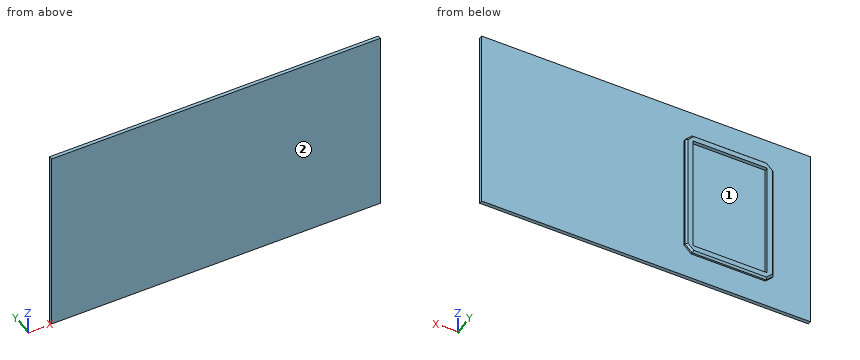
Autodesk Inventor part; units mm, degrees
ref_plane "YZ Plane" through (0, 0, 0) normal (1, 0, 0) x (0, 1, 0)
ref_plane "XZ Plane" through (0, 0, 0) normal (0, 1, 0) x (-1, 0, 0)
ref_plane "XY Plane" through (0, 0, 0) normal (0, 0, 1) x (1, 0, 0)
sketch "Sketch1" plane through (0, 0, 0) normal (0, 1, 0) x (-1, 0, 0)
  line L0 (0, 0) -> (-609.6, 0)
  line L1 (-609.6, 0) -> (-609.6, -342.9)
  line L2 (-609.6, -342.9) -> (0, -342.9)
  line L3 (0, -342.9) -> (0, 0)
  dimension "d0" = 609.6
  dimension "d1" = 342.9
  dimension "d2" = 609.6
extrude "Extrusion1" add sketch "Sketch1" along normal blind 6.35
sketch "Sketch2" plane through (0, 0, 0) normal (0, 1, 0) x (-1, 0, 0)
  line L0 (-609.6, -342.9) -> (0, -342.9)
  line L1 (0, 0) -> (-609.6, 0)
  line L2 (-609.6, -342.9) -> (-603.25, -342.9)
  line L3 (-603.25, -342.9) -> (-603.25, 0)
  line L4 (-603.25, 0) -> (-609.6, 0)
  line L5 (-609.6, 0) -> (-609.6, -342.9)
  dimension "d5" = 6.35
extrude "Extrusion2" cut sketch "Sketch2" along normal blind 231.775
sketch "Sketch3" plane through (0, 6.35, 0) normal (0, 1, 0) x (1, 0, 0)
  line L0 (603.25, 0) -> (603.25, 342.9)
  line L1 (0, 342.9) -> (0, 0)
  dimension "d8" = 603.25
sketch "Sketch4" plane through (0, 6.35, 0) normal (0, 1, 0) x (1, 0, 0)
  line L0 (603.25, 342.9) -> (0, 342.9)
  line L1 (0, 0) -> (603.25, 0)
  line L2 (0, 342.9) -> (0, 0)
  line L3 (0, 0) -> (301.625, 0)
  line L4 (301.625, 0) -> (301.625, 342.9)
  line L5 (301.625, 0) -> (452.4375, 0)
  line L6 (82.8675, 171.45) -> (82.8675, 280.162)
  line L7 (82.8675, 280.162) -> (150.8125, 280.162)
  line L8 (82.8675, 171.45) -> (82.8675, 62.738)
  line L9 (82.8675, 62.738) -> (150.8125, 62.738)
  line L10 (218.7575, 280.162) -> (150.8125, 280.162)
  line L11 (218.7575, 171.45) -> (218.7575, 280.162)
  line L12 (218.7575, 171.45) -> (218.7575, 62.738)
  line L13 (218.7575, 62.738) -> (150.8125, 62.738)
  line L14 (218.7575, 280.162) -> (218.7575, 292.862)
  line L15 (218.7575, 292.862) -> (82.8675, 292.862)
  line L16 (82.8675, 292.862) -> (82.8675, 280.162)
  line L17 (87.7385, 280.162) -> (75.0385, 280.162)
  line L18 (77.9965, 62.738) -> (87.7385, 62.738)
  line L19 (82.8675, 280.162) -> (70.1675, 280.162)
  line L20 (70.1675, 280.162) -> (70.1675, 62.738)
  line L21 (70.1675, 62.738) -> (82.8675, 62.738)
  line L22 (82.8675, 62.738) -> (82.8675, 50.038)
  line L23 (82.8675, 50.038) -> (218.7575, 50.038)
  line L24 (218.7575, 50.038) -> (218.7575, 62.738)
  line L25 (218.7575, 62.738) -> (231.4575, 62.738)
  line L26 (231.4575, 62.738) -> (231.4575, 280.162)
  line L27 (231.4575, 280.162) -> (218.7575, 280.162)
  line L28 (231.4575, 62.738) -> (218.7575, 50.038)
  line L29 (82.8675, 50.038) -> (70.1675, 62.738)
  line L30 (70.1675, 62.738) -> (70.1675, 280.162)
  line L31 (82.8675, 292.862) -> (70.1675, 280.162)
  line L32 (218.7575, 292.862) -> (231.4575, 280.162)
  dimension "d9" = 342.9
  dimension "d10" = 301.625
  dimension "d11" = 150.8125
extrude "Extrusion3" add sketch "Sketch4" along normal blind 6.35 contours L8 L18 L21 L20 L19 L17 L6 | L16 L15 L14 L10 L7 | L17 L19 L31 L16 | L22 L29 L21 L18 | L9 L13 L24 L23 L22 | L32 L27 L14 | L24 L25 L28 | L27 L26 L25 L12 L11
chamfer "Chamfer1" distance 3.175 angle 45 8 edges at (70.1675, 12.7, -171.45) (76.5175, 12.7, -286.512) (150.8125, 12.7, -292.862) (225.1075, 12.7, -286.512) (231.4575, 12.7, -171.45) (225.1075, 12.7, -56.388) (150.8125, 12.7, -50.038) (76.5175, 12.7, -56.388)
properties part number "UpperHalfofFrontBack_Ocampo"
Check sheet for the modelled part. Datum: model origin and axes. Units: mm. Face numbers are marked on the shaded views. A direction names the side the tool comes from. Coordinates: 2 decimals unless noted, no trailing zeros. Order: outer loops, then holes, each group sorted by start corner. A loop starts at its lowest first (then second) coordinate and runs counter-clockwise, first axis right, second up. Notation, with made-up numbers: (84, -8) -> (140, -8) arc R20 ccw to (140, -3) -> close; hole circle Ø8 at (-22.75, 75). An arc over 180 degrees is marked (long way). Write item = value, one per line. Start each with the question number.
1) Go/stop test with flat-tipped pins: P1, Ø2.5, axis at x = 175.5, y = 8, coming from the +Z side; P2, Ø3, axis at y = 9.5, z = -143.5, coming from the +X side; P3, Ø2.5, axis at y = 8, z = -119, coming from the -X side. Record where each tip stops, or that it passes through.
2) Cross-section at C-C (z = -314). Enter the section's corners in (x, y), then the cut area to 3 significant figures.
3) Cross-section at A-A (x = 110). Enter the section's corners in (y, z) (3 decimals).
4) Access from +Z, -Z, +X, -X, +Y, -Y to the whole of each face (thin tool, end or side, straight path). Record for the marked faces 1 and 2.
5) Material ranges on L1, parallel to X at y = 6.75, z = -164.5; L2, parallel to Y at x = 59.5, z = -94; L3, parallel to X at y = 11, z = -218.5, recorded low to high.
6) Cross-section at D-D (x = 342.5). Enter the section's corners in (y, z), then the cut area to 3 significant figures.
Ans:
q1.P1 = -50.04
q1.P2 = 231.46
q1.P3 = 70.17
q2.outline = (0, 0) -> (603.25, 0) -> (603.25, 6.35) -> (0, 6.35) -> close
q2.area = 3,830 mm²
q3.outline = (0, -342.9) -> (6.35, -342.9) -> (6.35, -292.862) -> (9.525, -292.862) -> (12.7, -289.687) -> (12.7, -280.162) -> (6.35, -280.162) -> (6.35, -62.738) -> (12.7, -62.738) -> (12.7, -53.213) -> (9.525, -50.038) -> (6.35, -50.038) -> (6.35, 0) -> (0, 0) -> close
q4.face_1 = +Y
q4.face_2 = +Z, -Z, +X, -X, -Y
q5.L1 = 70.17 to 82.87, 218.76 to 231.46
q5.L2 = 0 to 6.35
q5.L3 = 71.64 to 82.87, 218.76 to 229.98
q6.outline = (0, -342.9) -> (6.35, -342.9) -> (6.35, 0) -> (0, 0) -> close
q6.area = 2,180 mm²
